Verification items for the finished model (mm, model axes). Coordinates: 2 decimals unless noted, no trailing zeros. Order: outer loops, then holes, each group sorted by start corner. A loop starts at its lowest first (then second) coordinate and runs counter-clockwise, first axis right, second up. Notation, with made-up numbers: M -0.75,49.25 L 8.25,49.25 A16 ccw 8.25,71.25 Z; hole C 89.25,60 d8. An arc over 180 degrees is marked long. Return JSON: item names as keys, results as strings. Group by question number.
Q1. Section check B-B, the plane z = 6. Enter the section's corners in (x, y).
Q2. Go/stop test with a flat-tipped pin: pin 1 Ø3 at (x, y) = (0, -1.5) entering from -Z. Record where the tip stops, or that it passes through.
Q3. Thickness scan on probe 1 along Y at (x, z) = (0, 7); probe 2 along Y at (x, z) = (-0.6, 7); probe 3 along X at (y, z) = (-0.7, 3.5). Record the ranges inside material, lowest first.
Q4. Section check A-A, the plane x = 0. Enter the section's corners in (y, z), then the cut area to 3 significant figures.
Q5. Mould release check, pull along X, two halves, no side actions. Record for faces 1 (the face through (1, 1, 0)), 2 (the face through (-0.27, -1.22, 7.15)), 3 (the face through (-2.104, -1.236, 14.943)): pulls with the +X half, pulls with the -X half, needs draft (parallel to the pull), parting line crosses it, or undercut.
from build123d import *

# Parameters (mm, degrees)
F0_R     = 1.25
F1_DEPTH = 15
F2_SIZE  = 0.5
F3_R     = 0.2


with BuildPart() as f1:
    # F0 (on Top) → F1 (new body)
    with BuildSketch(Plane.XY):
        Polygon((1.443376, 2.5), (-1.443376, 2.5), (-2.886751, 0), (-1.443376, -2.5), (1.443376, -2.5), (2.886751, 0), align=None)
        Circle(F0_R, mode=Mode.SUBTRACT)
    extrude(amount=F1_DEPTH)

    # F2
    f2_edges = [f1.edges().sort_by_distance(p)[0] for p in [
        (-1.25, 0, 15),
    ]]
    chamfer(f2_edges, length=F2_SIZE)

    # F3
    f3_edges = [f1.edges().sort_by_distance(p)[0] for p in [
        (-2.165064, -1.25, 15),
        (0, -2.5, 15),
        (2.165064, -1.25, 15),
        (2.165064, 1.25, 15),
        (0, 2.5, 15),
        (-2.165064, 1.25, 15),
        (-2.165064, -1.25, 0),
        (0, -2.5, 0),
        (2.165064, -1.25, 0),
        (2.165064, 1.25, 0),
        (0, 2.5, 0),
        (-2.165064, 1.25, 0),
        (-1.443376, -2.5, 7.5),
        (1.443376, -2.5, 7.5),
        (-2.886751, 0, 7.5),
        (-1.443376, 2.5, 7.5),
        (1.443376, 2.5, 7.5),
        (2.886751, 0, 7.5),
    ]]
    fillet(f3_edges, radius=F3_R)


solid = f1.part
Numbers:
{
 "1": {"outline": "M -2.83,-0.1 L -1.5,-2.4 A0.2 ccw -1.33,-2.5 L 1.33,-2.5 A0.2 ccw 1.5,-2.4 L 2.83,-0.1 A0.2 ccw 2.83,0.1 L 1.5,2.4 A0.2 ccw 1.33,2.5 L -1.33,2.5 A0.2 ccw -1.5,2.4 L -2.83,0.1 A0.2 ccw Z; hole C 0,0 d2.5"},
 "2": {"pin 1": "stops at z = 0"},
 "3": {"probe 1": "y = -2.5 to -1.25, 1.25 to 2.5", "probe 2": "y = -2.5 to -1.1, 1.1 to 2.5", "probe 3": "x = -2.48 to -1.04, 1.04 to 2.48"},
 "4": {"outline": "M -2.5,0.2 A0.2 ccw -2.3,0 L -1.25,0 L -1.25,14.5 L -1.75,15 L -2.3,15 A0.2 ccw -2.5,14.8 Z; M 1.25,0 L 2.3,0 A0.2 ccw 2.5,0.2 L 2.5,14.8 A0.2 ccw 2.3,15 L 1.75,15 L 1.25,14.5 Z", "area": "37.2 mm2"},
 "5": {"face 1": "needs draft", "face 2": "undercut", "face 3": "pulls with the -X half"}
}
